from build123d import *

# Parameters (mm, degrees)
F0_R        = 1.75
F1_DEPTH    = 3
F2_W        = 50
F2_H        = 3
F2_H_2      = 27
F2_R        = 1
F2_R_2      = 1.5
F3_DEPTH    = 3
F4_T1_DEPTH = 53
F4_T3_DEPTH = 53
F4_T5_DEPTH = 50.6969600708
F5_R        = 5


# Not quite as in the source:
# - a fillet or chamfer that OpenCascade refuses, or shapes differently, is made with other operations: its cross-section is extruded or revolved along the edge and cut away or added


with BuildPart() as f1:
    # F0 (on Front) → F1 (new body)
    with BuildSketch(Plane.XZ):
        Polygon((-6, 20), (-25, 20), (-25, -20), (25, -20), (25, 20), (6, 20), (6, 13), (-6, 13), align=None)
        with Locations((-14.25, -13.75)):
            Circle(F0_R, mode=Mode.SUBTRACT)
        with Locations((14.25, -13.75)):
            Circle(F0_R, mode=Mode.SUBTRACT)
        with Locations((-14.25, 13.75)):
            Circle(F0_R, mode=Mode.SUBTRACT)
        with Locations((14.25, 13.75)):
            Circle(F0_R, mode=Mode.SUBTRACT)
    extrude(amount=F1_DEPTH)

    # F2 (on face) → F3 (join)
    with BuildSketch(Plane(origin=(0, 0, -20), x_dir=(1, 0, 0), z_dir=(0, 0, -1))):
        with Locations((0, 1.5)):
            Rectangle(F2_W, F2_H)
        with Locations((0, -13.5)):
            Rectangle(F2_W, F2_H_2)
        with Locations((-8.5, -12.5)):
            Circle(F2_R, mode=Mode.SUBTRACT)
        with Locations((0, -22.5)):
            Circle(F2_R, mode=Mode.SUBTRACT)
        with Locations((0, -12.5)):
            Circle(F2_R_2, mode=Mode.SUBTRACT)
        with Locations((8.5, -12.5)):
            Circle(F2_R, mode=Mode.SUBTRACT)
    extrude(amount=F3_DEPTH)

    # F4: fillet of radius 10 on 6 edges, made by hand

    # F4_s2 → F4_t1 (cut)
    with BuildSketch(Plane.XY.offset(-48)):
        with BuildLine():
            ThreePointArc((25, 17), (22.0710678119, 24.0710678119), (15, 27))
            Line((15, 27), (25, 27))
            Line((25, 27), (25, 17))
        make_face()
        with BuildLine():
            ThreePointArc((-15, 27), (-22.0710678119, 24.0710678119), (-25, 17))
            Line((-25, 17), (-25, 27))
            Line((-25, 27), (-15, 27))
        make_face()
    extrude(amount=F4_T1_DEPTH, mode=Mode.SUBTRACT)

    # F4_s4 → F4_t3 (cut)
    with BuildSketch(Plane.XZ.offset(-25)):
        with BuildLine():
            ThreePointArc((-15, 20), (-22.0710678119, 17.0710678119), (-25, 10))
            Line((-25, 10), (-25, 20))
            Line((-25, 20), (-15, 20))
        make_face()
        with BuildLine():
            ThreePointArc((15, 20), (22.0710678119, 17.0710678119), (25, 10))
            Line((25, 10), (25, 20))
            Line((25, 20), (15, 20))
        make_face()
    extrude(amount=F4_T3_DEPTH, mode=Mode.SUBTRACT)

    # F4_s6 → F4_t5 (cut)
    with BuildSketch(Plane.XZ.offset(-23.8484800354)):
        with BuildLine():
            ThreePointArc((6, 13), (9.6233122311, 18.0622577483), (15.5393920142, 20))
            Line((15.5393920142, 20), (6, 20))
            Line((6, 20), (6, 13))
        make_face()
        with BuildLine():
            ThreePointArc((-15.5393920142, 20), (-9.6233122311, 18.0622577483), (-6, 13))
            Line((-6, 13), (-6, 20))
            Line((-6, 20), (-15.5393920142, 20))
        make_face()
    extrude(amount=F4_T5_DEPTH, mode=Mode.SUBTRACT)

    # F5
    f5_edges = [f1.edges().sort_by_distance(p)[0] for p in [
        (6, -1.5, 13),
        (-6, -1.5, 13),
    ]]
    fillet(f5_edges, radius=F5_R)


solid = f1.part
The listing builds one solid part. Answer for the finished solid, in the listing's coordinates (mm). A direction names the side the tool comes from. Round coordinates to 2 decimals unless told otherwise and drop trailing zeros. Write each loop counter-clockwise with the first axis right and the second up, starting at its lowest first coordinate (ties: lowest second). Pieces come first, ordered by that corner, then holes. Notation, with made-up numbers: M 70.25,49 L 103.25,49 A19 cw 103.25,79 Z; hole C 61,71.5 d2. An arc over 180 degrees is marked long. Write each question's results on one line, items separated by ' | '. Start each with the question number.
(1) The part is cut by section C-C, the plane x = -8.5. Write down the section's boundary in (y, z).
(2) Determine the mould class of faces 1 (the flat face through (0, -1, 13)), 2 (the flat face through (0, 27, -21)), 3 (the flat face through (-25, -0.5, -10.1)), 4 (the cylindrical face through (22.09, -1.48, 17.05)) for opening direction X: +X half, -X half, draft (parallel to the pull), parting line (faces both ways), or undercut.
(3) Each of these flat-tipped pins is pushed along its axis until it touches: P1, Ø4, axis at x = 14.25, z = -13.75, coming from the +Y side; P2, Ø0.9, axis at x = 0, y = -2, coming from the +Z side; P3, Ø2.5, axis at x = 0, y = 12.5, coming from the +Z side; P4, Ø2.5, axis at x = 0, y = 22.5, coming from the +Z side. Where does it stop, or does it pass through?
(4) For faces 5 (the flat face through (0, 0, 0)), 6 (the cylindrical face through (7.7, 13.1, -21.5)), 7 (the cylindrical face through (-5.3, -1.52, 13.64)), determine the directions among +Z, -Z, +X, -X, +Y, -Y from which every point of the face is accessible in a straight line to the end or side of a thin tool.
(5) The part is cut by section B-B, the plane x = 14.25. Write down the section's boundary in (y, z), and give its area (3 significant figures).
(6) The part is cut by section A-A, the plane z = -13.75. Write down the section's boundary in (x, y), and give its area (3 significant figures).
(7) Find the intervals of material crossed by line 1 (X direction, y = 12.5, z = -22.1); line 2 (Z direction, x = -14.25, y = -0.9); line 3 (Y direction, x = -19.5, z = 5.5), in increasing order.
(8) The part is cut by section D-D, the plane z = 8.5. Write down the section's boundary in (x, y).
Worked answers:
1) outline: M -3,-23 L 11.5,-23 L 11.5,-20 L 0,-20 L 0,17.1 L -3,17.1 Z; M 13.5,-23 L 27,-23 L 27,-20 L 13.5,-20 Z
2) face 1: undercut | face 2: draft | face 3: -X half | face 4: +X half
3) P1: stops at y = 0 | P2: stops at z = 13 | P3: passes through | P4: stops at z = -20
4) face 5: +Z, +X, -X, +Y | face 6: +Z, -Z | face 7: +Z, +Y, -Y
5) outline: M -3,-23 L 27,-23 L 27,-20 L 0,-20 L 0,-15.5 L -3,-15.5 Z; M -3,-12 L 0,-12 L 0,12 L -3,12 Z; M -3,15.5 L 0,15.5 L 0,19.92 L -3,19.92 Z | area: 189 mm²
6) outline: M -25,-3 L -16,-3 L -16,0 L -25,0 Z; M -12.5,-3 L 12.5,-3 L 12.5,0 L -12.5,0 Z; M 16,-3 L 25,-3 L 25,0 L 16,0 Z | area: 129 mm²
7) line 1: x = -25 to -9.5, -7.5 to -1.5, 1.5 to 7.5, 9.5 to 25 | line 2: z = -23 to -15.5, -12 to 12, 15.5 to 19.92 | line 3: y = -3 to 0
8) outline: M -25,-3 L 25,-3 L 25,0 L -25,0 Z
